The listing builds one solid part. Answer for the finished solid, in the listing's coordinates (mm). Round coordinates to 2 decimals unless told otherwise and drop trailing zeros. Write each loop counter-clockwise with the first axis right and the second up, starting at its lowest first coordinate (ties: lowest second). Pieces come first, ordered by that corner, then holes. Notation, with made-up numbers: (83.5, 56) - (115.5, 56) arc R29 cw to (115.5, 81) - close; hole circle Ø3 at (89.5, 45). An arc over 180 degrees is marked (long way). Return JSON: item names as keys, results as strings. Group by question number.
(1) Section A-A, the plane z = 406.4 is taken. Write down the section's boundary in (x, y), then the cut area to 3 significant figures.
(2) Find the intervals of material crossed by line 1 along Z through (x, y) = (1, 88); line 2 along Z through (x, y) = (0.7, -41); line 3 along Y through (x, z) = (-1.35, -89), in increasing order. Write a range as [from, to].
(3) This flat-tipped pin is pushed along its axis until it touches: pin 1 (1 mm diameter, centred on x = -0.5, z = -466, fed in from -Y). Where does it stop, or does it pass through?
(4) Section C-C, the plane z = -383 is taken. Write down the section's boundary in (x, y), then the cut area to 3 significant figures.
(5) Section D-D, the plane x = 0.05 is taken. Give the number of separate pieces and of enclosed holes in the cut face, then the cut area to 3 significant figures.
(6) Section B-B, the plane y = 82.55 is taken. Write down the section's boundary in (x, z).
(7) Determine the mould class of faces 1 (the cylindrical face through (0.02, -30.92, -38.72)), 2 (the flat face through (-1.588, -12, 8)), 3 (the cylindrical face through (0.02, 75.94, 456.77)) for opening direction Y: +Y half, -Y half, draft (parallel to the pull), parting line (faces both ways), or undercut.
```python
from build123d import *

# Parameters (mm, degrees)
F0_W     = 1752.6
F0_H     = 1143
F1_DEPTH = 1.5875
F2_W     = 50.8
F2_H     = 215.9
F3_DEPTH = 3.176
F5_DEPTH = 3.176
F6_R     = 50.8
F7_DEPTH = 3.176
F9_DEPTH = 3.176
F10_R    = 5.08


with BuildPart() as f1:
    # F0 (on Right) → F1 (new body, symmetric)
    with BuildSketch(Plane.YZ):
        Rectangle(F0_W, F0_H)
    extrude(amount=F1_DEPTH, both=True)

    # F2 (on face) → F3 (cut, through all)
    with BuildSketch(Plane.YZ.offset(1.5875)):
        with Locations((-850.9, 412.75)):
            Rectangle(F2_W, F2_H)
        with Locations((850.9, 412.75)):
            Rectangle(F2_W, F2_H)
        with Locations((-850.9, -412.75)):
            Rectangle(F2_W, F2_H)
        with Locations((850.9, -412.75)):
            Rectangle(F2_W, F2_H)
    extrude(amount=-F3_DEPTH, mode=Mode.SUBTRACT)

    # F4 (on face) → F5 (cut, through all)
    with BuildSketch(Plane.YZ.offset(1.5875)):
        with BuildLine():
            Line((-269.875, 44.45), (-269.875, 146.05))
            ThreePointArc((-269.875, 146.05), (-288.925, 165.1), (-307.975, 146.05))
            Line((-307.975, 146.05), (-307.975, 44.45))
            ThreePointArc((-307.975, 44.45), (-288.925, 25.4), (-269.875, 44.45))
        make_face()
        with BuildLine():
            ThreePointArc((307.975, 146.05), (288.925, 165.1), (269.875, 146.05))
            Line((269.875, 146.05), (269.875, 44.45))
            ThreePointArc((269.875, 44.45), (288.925, 25.4), (307.975, 44.45))
            Line((307.975, 44.45), (307.975, 146.05))
        make_face()
    extrude(amount=-F5_DEPTH, mode=Mode.SUBTRACT)

    # F6 (on face) → F7 (cut, through all)
    with BuildSketch(Plane.YZ.offset(1.5875)):
        with Locations((82.55, 406.4)):
            Circle(F6_R)
        with Locations((-79.375, -53.975)):
            Circle(F6_R)
    extrude(amount=-F7_DEPTH, mode=Mode.SUBTRACT)

    # F8 (on face) → F9 (cut, through all)
    with BuildSketch(Plane.YZ.offset(1.5875)):
        Polygon((-101.6, -539.75), (-130.175, -571.5), (130.175, -571.5), (101.6, -539.75), align=None)
    extrude(amount=-F9_DEPTH, mode=Mode.SUBTRACT)

    # F10
    f10_edges = [f1.edges().sort_by_distance(p)[0] for p in [
        (0, -876.3, -571.5),
        (0, -876.3, -520.7),
        (0, -876.3, -304.8),
        (0, -876.3, 304.8),
        (0, -876.3, 520.7),
        (0, -876.3, 571.5),
        (0, 876.3, 571.5),
        (0, 876.3, 520.7),
        (0, 876.3, 304.8),
        (0, 876.3, -304.8),
        (0, 876.3, -520.7),
        (0, 876.3, -571.5),
        (0, 130.175, -571.5),
        (0, -130.175, -571.5),
        (0, -101.6, -539.75),
        (0, 101.6, -539.75),
    ]]
    fillet(f10_edges, radius=F10_R)


solid = f1.part
```
Working result:
{
 "1": {"outline": "(-1.59, -825.5) - (1.59, -825.5) - (1.59, 31.75) - (-1.59, 31.75) - close; (-1.59, 133.35) - (1.59, 133.35) - (1.59, 825.5) - (-1.59, 825.5) - close", "area": "4,920 mm^2"},
 "2": {"line 1": "z = [-539.75, 355.89], [456.91, 571.5]", "line 2": "z = [-539.75, -87.26], [-20.69, 571.5]", "line 3": "y = [-876.3, -116.17], [-42.58, 876.3]"},
 "3": {"pin 1": "stops at y = -825.5"},
 "4": {"outline": "(-1.59, -825.5) - (1.59, -825.5) - (1.59, 825.5) - (-1.59, 825.5) - close", "area": "5,240 mm^2"},
 "5": {"separate pieces": "1", "enclosed holes": "4", "area": "1,930,000 mm^2"},
 "6": {"outline": "(-1.59, -539.75) - (1.59, -539.75) - (1.59, 355.6) - (-1.59, 355.6) - close; (-1.59, 457.2) - (1.59, 457.2) - (1.59, 571.5) - (-1.59, 571.5) - close"},
 "7": {"face 1": "undercut", "face 2": "draft", "face 3": "undercut"}
}
